Input: part model. Units: mm. Frame: model coordinates. A direction names the side the tool comes from. Coordinates: 2 decimals unless noted, no trailing zeros. Write each loop counter-clockwise with the first axis right and the second up, starting at its lowest first coordinate (ties: lowest second). Pieces come first, ordered by that corner, then holes. Notation, with made-up numbers: (-24, -13) - (16, -13) arc R37 cw to (16, 24) - close; hole circle Ø10 at (54, 36). An arc over 180 degrees is marked (long way). Use a Markdown table: item, result. Add a question column.
Q1. Section query A-A (x = 91). Return the cut outline in (y, z).
Q2. Section query B-B (y = 1.8). Give the number of separate pieces and of enclosed holes in the cut face, then the cut area to 3 significant figures.
Q3. Material intervals for probe 1 along Z at (x, y) = (-90.5, 0.45); probe 2 along X at (y, z) = (2.9, 12); probe 3 along Z at (x, y) = (108, 1.45), sorted ascending. Write a range as from..to.
Q4. Section query C-C (z = 35.5). Return the cut outline in (x, y).
Q5. Mould query, pull axis X, two halves, no side actions, for faces 3 (the face through (0, 2, -8.352)), 4 (the face through (7.811, 2, 14)), 5 (the face through (-2, 2, -14.785)), 6 (the face through (-120, 2, 16)). Classes: released by +X, released by -X, zero draft, split by the parting line, or undercut.
Q6. Set-up query: faces 1 (the face through (-2, 0, 8)), 2 (the face through (0, 2, 11.648)). Return all of +Z, -Z, +X, -X, +Y, -Y with unobstructed straight access to the full face (end or side cutting, diameter ignored); none if empty.
from build123d import *

# Parameters (mm, degrees)
SKETCH1_W           = 240
SKETCH1_H           = 60
SKETCH1_R           = 5.248248104
SKETCH1_R_2         = 1.5
SKETCH1_R_3         = 2.75
SKETCH1_R_4         = 2.5
SKETCH1_W_2         = 15
SKETCH1_H_2         = 5
BOSS_EXTRUDE1_DEPTH = 5


with BuildPart() as part:
    # Sketch1 → Boss-Extrude1 (new body)
    with BuildSketch(Plane(origin=(0, 0, 0), x_dir=(1, 0, 0), z_dir=(0, 1, 0))):
        with Locations((0, -15.214636322)):
            Rectangle(SKETCH1_W, SKETCH1_H)
        with Locations(Location((-91, -35.214636322, 0), (0, 0, 270))):
            Circle(SKETCH1_R, mode=Mode.SUBTRACT)
        with Locations(Location((91, -35.214636322, 0), (0, 0, 90))):
            Circle(SKETCH1_R, mode=Mode.SUBTRACT)
        with Locations(Location((-110, -0.214636322, 0), (0, 0, 270))):
            Circle(SKETCH1_R_2, mode=Mode.SUBTRACT)
        with Locations(Location((110, -0.214636322, 0), (0, 0, 270))):
            Circle(SKETCH1_R_2, mode=Mode.SUBTRACT)
        with Locations(Location((-74.75, -35.214636322, 0), (0, 0, 270))):
            Circle(SKETCH1_R_3, mode=Mode.SUBTRACT)
        with Locations(Location((-107.25, -35.214636322, 0), (0, 0, 270))):
            Circle(SKETCH1_R_3, mode=Mode.SUBTRACT)
        with Locations(Location((107.25, -35.214636322, 0), (0, 0, 270))):
            Circle(SKETCH1_R_3, mode=Mode.SUBTRACT)
        with Locations(Location((75, -35.214636322, 0), (0, 0, 270))):
            Circle(SKETCH1_R_4, mode=Mode.SUBTRACT)
        with Locations((0.310691637, -14.147905604)):
            Rectangle(SKETCH1_W_2, SKETCH1_H_2, mode=Mode.SUBTRACT)
        with Locations((0, 10.852094396)):
            Rectangle(SKETCH1_W_2, SKETCH1_H_2, mode=Mode.SUBTRACT)
    extrude(amount=BOSS_EXTRUDE1_DEPTH)


solid = part.part
Values follow:
| question | item | result |
|---|---|---|
| 1 | outline | (0, -14.79) - (5, -14.79) - (5, 29.97) - (0, 29.97) - close; (0, 40.46) - (5, 40.46) - (5, 45.21) - (0, 45.21) - close |
| 2 | separate pieces | 1 |
| 2 | enclosed holes | 10 |
| 2 | area | 14,000 mm2 |
| 3 | probe 1 | -14.79..29.99, 40.44..45.21 |
| 3 | probe 2 | -120..-7.19, 7.81..120 |
| 3 | probe 3 | -14.79..32.57, 37.86..45.21 |
| 4 | outline | (-120, 0) - (-109.99, 0) - (-109.99, 5) - (-120, 5) - close; (-104.51, 0) - (-96.24, 0) - (-96.24, 5) - (-104.51, 5) - close; (-85.76, 0) - (-77.49, 0) - (-77.49, 5) - (-85.76, 5) - close; (-72.01, 0) - (72.52, 0) - (72.52, 5) - (-72.01, 5) - close; (77.48, 0) - (85.76, 0) - (85.76, 5) - (77.48, 5) - close; (96.24, 0) - (104.51, 0) - (104.51, 5) - (96.24, 5) - close; (109.99, 0) - (120, 0) - (120, 5) - (109.99, 5) - close |
| 5 | face 3 | undercut |
| 5 | face 4 | undercut |
| 5 | face 5 | zero draft |
| 5 | face 6 | released by -X |
| 6 | face 1 | +Z, -Z, +X, -X, -Y |
| 6 | face 2 | +Y, -Y |
